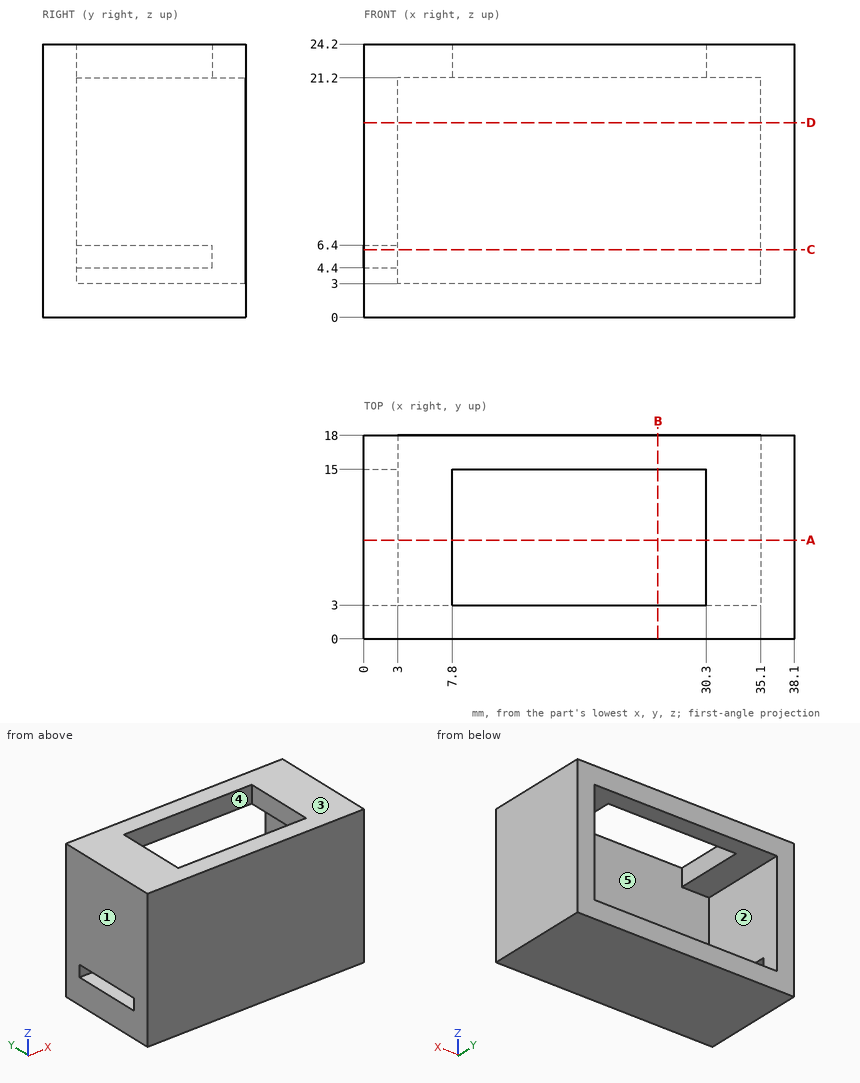
Job drawing, mm, ordinate dimensions from the low corner. One solid piece. A direction names the side the tool comes from. Give positions to 0.01 mm unless a question says otherwise; leave off trailing zeros. Loops run counter-clockwise (first coordinate to the right, second up) from the corner with the lowest first, then second, coordinate; pieces in that order, holes last. Notation, with made-up numbers: M -10.5,69 L 25.5,69 A28 cw 25.5,102 Z; hole C 62.25,27.5 d3. An arc over 180 degrees is marked long. Use one line per item in the form item = value.
Item 1: Slice it at D-D on z = 17.25. List the corners of the cut face in (x, y).
Filled in:
outline = M 0,0 L 38.1,0 L 38.1,18 L 35.1,18 L 35.1,3 L 3,3 L 3,18 L 0,18 Z
Item 2: Slice it at B-B on x = 26. List the corners of the cut face in (y, z), and give its area (3 significant figures).
Filled in:
outline = M 0,0 L 18,0 L 18,3 L 3,3 L 3,24.2 L 0,24.2 Z; M 15,21.2 L 18,21.2 L 18,24.2 L 15,24.2 Z
area = 127 mm^2
Item 3: Slice it at A-A on y = 8.75. List the corners of the cut face in (x, z), and give its area (3 significant figures).
Filled in:
outline = M 0,0 L 38.1,0 L 38.1,24.2 L 30.3,24.2 L 30.3,21.2 L 35.1,21.2 L 35.1,3 L 3,3 L 3,4.4 L 0,4.4 Z; M 0,6.4 L 3,6.4 L 3,21.2 L 7.8,21.2 L 7.8,24.2 L 0,24.2 Z
area = 264 mm^2
Item 4: Flat gauge pins, fed straight in: pin 1 Ø2 at (x, z) = (8.5, 6) entering from +Y; pin 2 Ø4.5 at (x, y) = (16.5, 7.5) entering from +Z. Where does each tip first touch, or does it go through?
Filled in:
pin_1 = 3
pin_2 = 3
Item 5: Drill centre lines: L1, parallel to Z at x = 5, y = 5.75; L2, parallel to X at y = 6, z = 19.5; L3, parallel to X at y = 8, z = 23. Where is each one in solid material? Low to high.
Filled in:
L1 = 0 to 3, 21.2 to 24.2
L2 = 0 to 3, 35.1 to 38.1
L3 = 0 to 7.8, 30.3 to 38.1
Item 6: Which spindle directions (+Z, -Z, +X, -X, +Y, -Y) get a long thin tool onto all of the face, cutting with end or side? Do the marked faces 1 and 2. Say none if no direction does.
Filled in:
face_1 = +Z, -Z, -X, +Y, -Y
face_2 = +Y
Item 7: Slice it at C-C on z = 6. List the corners of the cut face in (x, y).
Filled in:
outline = M 0,0 L 38.1,0 L 38.1,18 L 35.1,18 L 35.1,3 L 0,3 Z; M 0,15 L 3,15 L 3,18 L 0,18 Z
Item 8: Two-plate mould, pull along Z, no slides. Class the marked faces 3, 4 and 5: released by +Z, released by -Z, zero draft, split by the parting line, or undercut.
Filled in:
face_3 = released by +Z
face_4 = zero draft
face_5 = undercut
